For this review, take the finished solid that the model builds, in its own axes (mm). A direction names the side the tool comes from. Coordinates: 2 decimals unless noted, no trailing zeros. Loops run counter-clockwise (first coordinate to the right, second up) from the corner with the lowest first, then second, coordinate; pieces in that order, holes last. Notation, with made-up numbers: (5, 82) - (19, 82) arc R10 ccw to (19, 86) - close; hole circle Ø8 at (-22.5, -2.5). An arc over 180 degrees is marked (long way). One line per item, written item: value. Start each with the question number.
1. Take a section at D-D, the plane y = -41.5. State the section outline as (x, z) points, and give its area (3 significant figures).
2. For faces 1 (the face through (11.6, -43.5, 0)), 2 (the face through (12.53, -41, -4)), 3 (the face through (16, -41, -6.3)), list the 3-axis set-ups (+Z, -Z, +X, -X, +Y, -Y) from which the entire face can be reached by the end or side of a thin tool; tool diameter is ignored.
3. Insertion check: pin 1 (1 mm diameter, centred on x = 9.5, z = -3.5, fed in from +Y); pin 2 (1 mm diameter, centred on x = 10.5, z = -6, fed in from -Y); pin 3 (2.5 mm diameter, centred on y = -41, z = -5.5, fed in from -X). Each pin has a flat end and moves straight along its axis. Give the tip position at first contact, or say it passes through.
4. Take a section at C-C, the plane x = 16. State the section outline as (y, z) points, and give its area (3 significant figures).
5. The part is to be moulded in two halves that separate along X. For faces 4 (the face through (19.13, -41, -4)), 5 (the face through (11.6, -43.5, -7.8)), 6 (the face through (15.82, -41.732, -3.934)), 7 (the face through (16, -41, -1.5)), say which applies: released by +X, released by -X, zero draft, split by the parting line, or undercut.
6. Take a section at B-B, the plane y = -40.25. State the section outline as (x, z) points.
7. Take a section at A-A, the plane z = -5.5. State the section outline as (x, y) points.
8. To check wall thickness, follow line 1 (Z direction, x = 8.5, y = -43); line 2 (X direction, y = -41.75, z = -6.5); line 3 (Y direction, x = 8, z = -1). State the ranges of each line that lie inside material, in increasing order. Write a range as from..to.
```python
from build123d import *

# Parameters (mm, degrees)
BOSS_EXTRUDE1_DEPTH = 7.8
SHELL1_START        = -6.3
SHELL1_DEPTH        = 4.8


# Read off the part's stored shape, not the designer's step: Shell1
with BuildPart() as part:
    # Sketch1 → Boss-Extrude1 (new body)
    with BuildSketch(Plane.XY):
        with BuildLine():
            Line((19.130275644, -41.976412541), (19.130275644, -39.726412541))
            Line((19.130275644, -39.726412541), (12.530275644, -39.726412541))
            Line((12.530275644, -39.726412541), (12.530275644, -42.926412541))
            Line((12.530275644, -42.926412541), (4.330275644, -42.926412541))
            Line((4.330275644, -42.926412541), (4.330275644, -45.926412541))
            ThreePointArc((4.330275644, -45.926412541), (11.895376904, -44.570019793), (19.130275644, -41.976412541))
        make_face()
    extrude(amount=-BOSS_EXTRUDE1_DEPTH)

    # Shell1 outline → Shell1 (cut)
    with BuildSketch(Plane.XY.offset(SHELL1_START)):
        with BuildLine():
            Line((14.030275644, -39.726412541), (14.030275644, -42.367413234))
            ThreePointArc((14.030275644, -42.367413234), (15.845028157, -41.722672751), (17.630275644, -41.000240481))
            Line((17.630275644, -41.000240481), (17.630275644, -39.726412541))
            Line((17.630275644, -39.726412541), (14.030275644, -39.726412541))
        make_face()
        with BuildLine():
            Line((5.830275644, -42.926412541), (5.830275644, -44.247646544))
            ThreePointArc((5.830275644, -44.247646544), (9.046039137, -43.703724266), (12.213494388, -42.926412541))
            Line((12.213494388, -42.926412541), (5.830275644, -42.926412541))
        make_face()
    extrude(amount=SHELL1_DEPTH, mode=Mode.SUBTRACT)


solid = part.part
```
Solutions:
1. outline: (12.53, -7.8) - (19.13, -7.8) - (19.13, 0) - (12.53, 0) - close; hole (14.03, -6.3) - (16.42, -6.3) - (16.42, -1.5) - (14.03, -1.5) - close
1. area: 40.0 mm2
2. face 1: +Z, +X, -X, +Y, -Y
2. face 2: +Z, -Z, -X, +Y
2. face 3: +Y
3. pin 1: y = -43.5
3. pin 2: y = -45.03
3. pin 3: x = 12.53
4. outline: (-43.27, -7.8) - (-39.73, -7.8) - (-39.73, -6.3) - (-41.66, -6.3) - (-41.66, -1.5) - (-39.73, -1.5) - (-39.73, 0) - (-43.27, 0) - close
4. area: 18.3 mm2
5. face 4: released by +X
5. face 5: zero draft
5. face 6: undercut
5. face 7: undercut
6. outline: (12.53, -7.8) - (19.13, -7.8) - (19.13, 0) - (12.53, 0) - close; hole (14.03, -6.3) - (17.63, -6.3) - (17.63, -1.5) - (14.03, -1.5) - close
7. outline: (4.33, -45.93) arc R46.13 ccw to (19.13, -41.98) - (19.13, -39.73) - (17.63, -39.73) - (17.63, -41) arc R44.63 cw to (14.03, -42.37) - (14.03, -39.73) - (12.53, -39.73) - (12.53, -42.93) - (12.21, -42.93) arc R44.63 cw to (5.83, -44.25) - (5.83, -42.93) - (4.33, -42.93) - close
8. line 1: -7.8..-6.3, -1.5..0
8. line 2: 12.53..19.13
8. line 3: -45.43..-42.93
